The model under review builds one solid part; all positions refer to its coordinate system, in mm. A direction names the side the tool comes from. Round coordinates to 2 decimals unless told otherwise and drop trailing zeros. Write each loop counter-clockwise with the first axis right and the second up, starting at its lowest first coordinate (ties: lowest second). Pieces come first, ordered by that corner, then holes.
Item 1: Clearance check with flat-ended pins moving along their axes: pin 1 Ø5 at (x, z) = (-8.5, -3) entering from +Y; pin 2 Ø1.5 at (x, y) = (-6.5, -9) entering from -Z; pin 3 Ø1.6 at (x, y) = (0, 0) entering from -Z; pin 4 Ø4 at (y, z) = (-4.5, -3.5) entering from +X. State where each tip first meets the part, or that it passes through.
Item 2: Add section C-C (y = -5). Give the boundary of the cut face in (x, z).
Item 3: Add section B-B (z = -12.5). Give the boundary of the cut face in (x, y), plus the area to 3 significant figures.
Item 4: Add section A-A (x = 0). Give the boundary of the cut face in (y, z), plus the area to 3 significant figures.
Item 5: To check wall thickness, follow L1, parallel to Y at x = 0, z = -12.25; L2, parallel to Y at x = 0, z = 2.8; L3, parallel to Z at x = 8.5, y = -5.75. State the ranges of each line that lie inside material, in increasing order.
Item 6: Add section D-D (x = 8.75). Give the boundary of the cut face in (y, z), plus the area to 3 significant figures.
Item 7: Machinability: for faces 1 (the face through (-1, 1, 5.5)), 2 (the face through (-0.158, -4.247, -23.746)), 3 (the face through (4.38, 8.43, 1.73)), which of the approach directions +Z, -Z, +X, -X, +Y, -Y give a long, thin tool a straight path to every point of the face, cutting with its end or side? Answer none if there is none.
Autodesk Inventor part; units mm, degrees
ref_plane "YZ Plane" through (0, 0, 0) normal (1, 0, 0) x (0, 1, 0)
ref_plane "XZ Plane" through (0, 0, 0) normal (0, 1, 0) x (-1, 0, 0)
ref_plane "XY Plane" through (0, 0, 0) normal (0, 0, 1) x (1, 0, 0)
sketch "basescetch" plane through (0, 0, 0) normal (0, 0, 1) x (1, 0, 0)
  circle A0 centre (0, 0) radius 11.85
  circle A1 centre (0, 0) radius 9.5
  circle A2 centre (0, 0) radius 3
  circle A3 centre (0, 0) radius 1
  dimension "d0" = 23.7
  dimension "d1" = 19
  dimension "d2" = 6
  dimension "d3" = 2
extrude "押し出し1" add sketch "basescetch" along normal blind 3.5 contours A1
extrude "押し出し2" add sketch "basescetch" along normal blind 5.5 contours A2
extrude "押し出し3" add sketch "basescetch" against normal blind 23.5 contours A0 | A1 | A2 | A3
sketch "スケッチ2" plane through (0, 0, -23.5) normal (0, 0, -1) x (-1, 0, 0)
  circle A0 centre (0, 0) radius 1
  arc A1 (-2, 3.75) -> (2, 3.75) centre (0, 0) ccw
  line L0 (0, -4.25) -> (0, -1)
  line L1 (0, -4.25) -> (8, -4.25) construction
  line L2 (0, 3.75) -> (2, 3.75)
  line L3 (-2, 3.75) -> (0, 3.75)
  dimension "d10" = 8.5
  dimension "d11" = 8
  dimension "d12" = 90
extrude "押し出し4" add sketch "スケッチ2" along normal blind 0.5
extrude "押し出し5" cut sketch "basescetch" against normal through all contours A3
properties part number "motor_for6speedgearbox" material "鉄、可鍛鉄"
Numbers:
1. pin 1: stops at y = 10.22
1. pin 2: stops at z = -23.5
1. pin 3: passes through
1. pin 4: stops at x = 11.58
2. outline: (-10.74, -23.5) - (10.74, -23.5) - (10.74, 0) - (8.08, 0) - (8.08, 3.5) - (-8.08, 3.5) - (-8.08, 0) - (-10.74, 0) - close
3. outline: circle Ø23.7 at (0, 0); hole circle Ø2 at (0, 0)
3. area: 438 mm2
4. outline: (-11.85, -23.5) - (-4.25, -23.5) - (-4.25, -24) - (-1, -24) - (-1, 5.5) - (-3, 5.5) - (-3, 3.5) - (-9.5, 3.5) - (-9.5, 0) - (-11.85, 0) - close; (1, -24) - (3.75, -24) - (3.75, -23.5) - (11.85, -23.5) - (11.85, 0) - (9.5, 0) - (9.5, 3.5) - (3, 3.5) - (3, 5.5) - (1, 5.5) - close
4. area: 580 mm2
5. L1: y = -11.85 to -1, 1 to 11.85
5. L2: y = -9.5 to -1, 1 to 9.5
5. L3: z = -23.5 to 0
6. outline: (-7.99, -23.5) - (7.99, -23.5) - (7.99, 0) - (3.7, 0) - (3.7, 3.5) - (-3.7, 3.5) - (-3.7, 0) - (-7.99, 0) - close
6. area: 401 mm2
7. face 1: +Z, +X, -X, +Y, -Y
7. face 2: -Z
7. face 3: +Z
